The model under review builds one solid part; all positions refer to its coordinate system, in mm. A direction names the side the tool comes from. Round coordinates to 2 decimals unless told otherwise and drop trailing zeros. Order: outer loops, then holes, each group sorted by start corner. A loop starts at its lowest first (then second) coordinate and runs counter-clockwise, first axis right, second up. Notation, with made-up numbers: (-10, 27) - (44, 27) arc R12 cw to (44, 34) - close; hole circle Ø10 at (10.25, -17.75). An arc over 180 degrees is marked (long way). One line per question, with ' | ' between items. Start each with the question number.
Item 1: Add section C-C on z = 0. State the section outline as (x, y) points.
Item 2: Tool access review of faces 4 (the face through (-13.516, -1, -4)), 5 (the face through (-5.973, -3.079, -0.087)): name each direction out of +Z, -Z, +X, -X, +Y, -Y from which nothing blocks a thin tool from reaching the whole face with its end or side.
Item 3: Add section A-A on y = 0. State the section outline as (x, z) points, and give its area (3 significant figures).
Item 4: Add section B-B on x = -5.5. State the section outline as (y, z) points.
Item 5: Draft analysis for pull direction Y (two halves, no side actions). For faces 1 (the face through (0, 2, 1)), 2 (the face through (-6.556, -2.055, -0.09)), 3 (the face through (-14.092, -0.853, 3.843)), state which applies: +Y half, -Y half, draft (parallel to the pull), parting line (faces both ways), or undercut.
Item 6: Add section D-D on x = -7. State the section outline as (y, z) points, and give its area (3 significant figures).
Item 7: Insertion check: pin 1 Ø2 at (y, z) = (1, 1) entering from -X; pin 2 Ø1.5 at (x, z) = (-6.5, -1) entering from -Y; pin 3 Ø4 at (x, z) = (-3, -3) entering from -Y. Each pin has a flat end and moves straight along its axis. Give the tip position at first contact, or say it passes through.
Item 8: For L1, parallel to Y at x = -7, z = 0; L2, parallel to Y at x = -10.75, z = -0.75, list the stretches that pass through material, from the lowest coordinate up. Write a range as [from, to].
from build123d import *

# Parameters (mm, degrees)
SKETCH2_R               = 1.984375
CUT_EXTRUDE1_DEPTH      = 5.7371001
CUT_EXTRUDE1_DEPTH_BACK = 5.7371001


with BuildPart() as part:
    # Sketch1 → Revolve1 (revolve)
    with BuildSketch(Plane.XY):
        with BuildLine():
            Line((0, 2.0574), (-12.931775, 2.0574))
            Line((-12.931775, 2.0574), (-14.684375, 3.81))
            Line((-14.684375, 3.81), (-14.684375, 3.937))
            Line((-14.684375, 3.937), (-13.515975, 3.937))
            Line((-13.515975, 3.937), (-13.515975, 4.7371))
            Line((-13.515975, 4.7371), (-0.381, 4.7371))
            ThreePointArc((-0.381, 4.7371), (-0.111592316, 4.625507684), (0, 4.3561))
            Line((0, 4.3561), (0, 2.0574))
        make_face()
    revolve(axis=Axis((0, 0, 0), (-1, 0, 0)))

    # Sketch2 → Cut-Extrude1 (cut, two sides)
    with BuildSketch(Plane(origin=(0, 0, 0), x_dir=(1, 0, 0), z_dir=(0, 1, 0))) as cut_extrude1_sk:
        with Locations((-3.990975, 0)):
            Circle(SKETCH2_R)
    extrude(amount=CUT_EXTRUDE1_DEPTH, mode=Mode.SUBTRACT)
    extrude(cut_extrude1_sk.sketch, amount=-CUT_EXTRUDE1_DEPTH_BACK, mode=Mode.SUBTRACT)


solid = part.part
Determined:
1) outline: (-14.68, -3.94) - (-13.52, -3.94) - (-13.52, -4.74) - (-5.98, -4.74) - (-5.98, -2.06) - (-12.93, -2.06) - (-14.68, -3.81) - close; (-14.68, 3.81) - (-12.93, 2.06) - (-5.98, 2.06) - (-5.98, 4.74) - (-13.52, 4.74) - (-13.52, 3.94) - (-14.68, 3.94) - close; (-2.01, -4.74) - (-0.38, -4.74) arc R0.38 ccw to (0, -4.36) - (0, -2.06) - (-2.01, -2.06) - close; (-2.01, 2.06) - (0, 2.06) - (0, 4.36) arc R0.38 ccw to (-0.38, 4.74) - (-2.01, 4.74) - close
2) face 4: -X | face 5: +Y, -Y
3) outline: (-14.68, -3.94) - (-13.52, -3.94) - (-13.52, -4.74) - (-0.38, -4.74) arc R0.38 ccw to (0, -4.36) - (0, -2.06) - (-12.93, -2.06) - (-14.68, -3.81) - close; (-14.68, 3.81) - (-12.93, 2.06) - (0, 2.06) - (0, 4.36) arc R0.38 ccw to (-0.38, 4.74) - (-13.52, 4.74) - (-13.52, 3.94) - (-14.68, 3.94) - close | area: 73.7 mm2
4) outline: (-4.56, -1.29) arc R4.74 ccw to (4.56, -1.29) - (1.6, -1.29) arc R2.06 cw to (-1.6, -1.29) - close; (-4.56, 1.29) - (-1.6, 1.29) arc R2.06 cw to (1.6, 1.29) - (4.56, 1.29) arc R4.74 ccw to start
5) face 1: draft | face 2: undercut | face 3: parting line
6) outline: circle Ø9.47 at (0, 0); hole circle Ø4.11 at (0, 0) | area: 57.2 mm2
7) pin 1: x = -13.29 | pin 2: y = -4.73 | pin 3: y = -4.61
8) L1: [-4.74, -2.06], [2.06, 4.74] | L2: [-4.68, -1.92], [1.92, 4.68]
